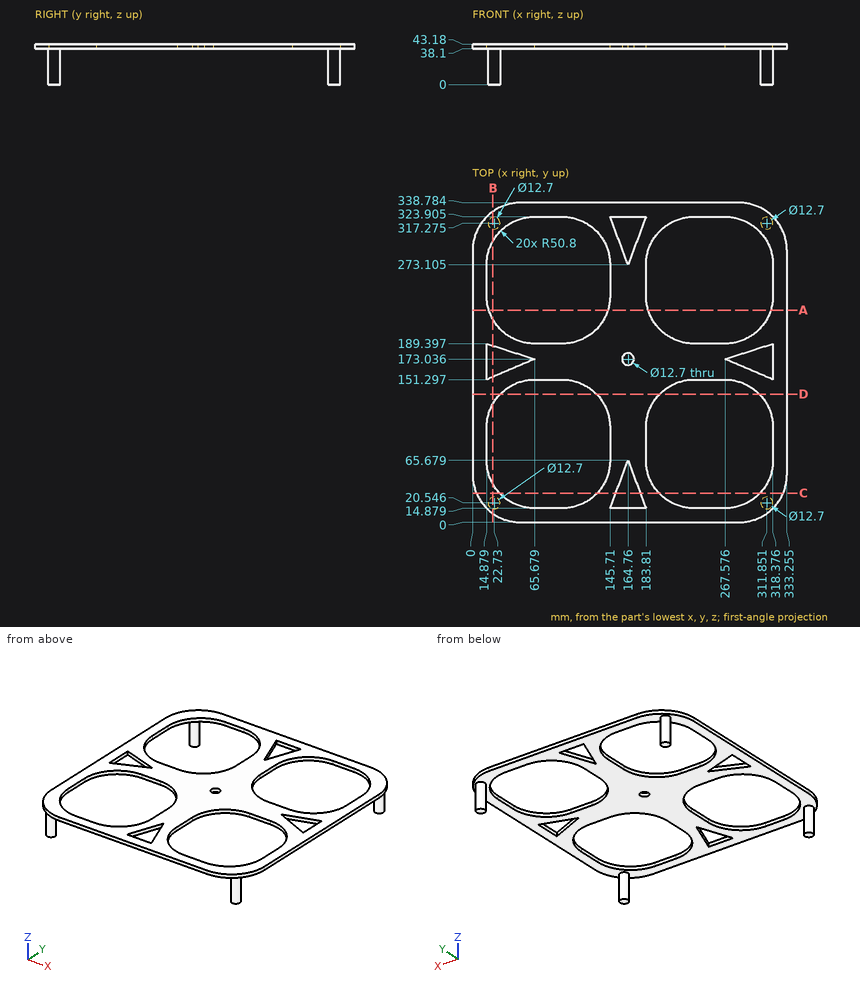
Here's the drawing with two shaded views (mm, measured from the low corner). I have some questions. Round coordinates to 2 decimals unless told otherwise and drop trailing zeros. Order: outer loops, then holes, each group sorted by start corner. A loop starts at its lowest first (then second) coordinate and runs counter-clockwise, first axis right, second up. Notation, with made-up numbers: (-4, 81.25) -> (12, 81.25) arc R14 ccw to (12, 101.25) -> close; hole circle Ø11 at (12.5, -13.75). An arc over 180 degrees is marked (long way). Use a Markdown table: item, result. Add a question column.
(1) I need wall thicknesses on line 1 along Y through (x, z) = (85.5, 40) (1 decimal); line 2 along Y through (x, z) = (300, 41) (1 decimal); line 3 along Z through (x, y) = (179, 100). Which ranges of each line are inside material? Lowest first, please.
(2) For pin 1 Ø6 at (x, y) = (187, 84.5) entering from -Z; pin 2 Ø4 at (x, y) = (250, 161.5) entering from -Z, each with a flat end and sliding along its axis, tell me the tip position at first contact or that it passes through.
(3) Suppose I cut it at A-A, the plane y = 225. Count the separate pieces of the cut face and the enclosed holes in it, and give its area (3 significant figures).
(4) Suppose I cut it at C-C, the plane y = 31. Please give me the cut outline in (x, z) (1 decimal).
(5) Suppose I cut it at D-D, the plane y = 136. Please give me the cut outline in (x, z) (1 decimal).
(6) Suppose I cut it at B-B, the plane x = 21.5. Please give me the cut outline in (y, z) (1 decimal).
Verdict:
| question | item | result |
|---|---|---|
| 1 | line 1 | 0 to 14.9, 151.3 to 189.4, 323.9 to 338.8 |
| 1 | line 2 | 3.1 to 26.6, 139.6 to 159.2, 183.5 to 201.1, 312.2 to 335.7 |
| 1 | line 3 | 38.1 to 43.18 |
| 2 | pin 1 | through |
| 2 | pin 2 | z = 38.1 |
| 3 | separate pieces | 3 |
| 3 | enclosed holes | 0 |
| 3 | area | 392 mm2 |
| 4 | outline | (4, 38.1) -> (28.6, 38.1) -> (28.6, 43.2) -> (4, 43.2) -> close; (132, 38.1) -> (151.8, 38.1) -> (151.8, 43.2) -> (132, 43.2) -> close; (177.8, 38.1) -> (197.5, 38.1) -> (197.5, 43.2) -> (177.8, 43.2) -> close; (304.7, 38.1) -> (329.2, 38.1) -> (329.2, 43.2) -> (304.7, 43.2) -> close |
| 5 | outline | (0, 38.1) -> (29.3, 38.1) -> (29.3, 43.2) -> (0, 43.2) -> close; (131.2, 38.1) -> (198.3, 38.1) -> (198.3, 43.2) -> (131.2, 43.2) -> close; (303.9, 38.1) -> (333.3, 38.1) -> (333.3, 43.2) -> (303.9, 43.2) -> close |
| 6 | outline | (9.3, 38.1) -> (14.3, 38.1) -> (14.3, 0) -> (26.8, 0) -> (26.8, 38.1) -> (40.6, 38.1) -> (40.6, 43.2) -> (9.3, 43.2) -> close; (125.6, 38.1) -> (154.1, 38.1) -> (154.1, 43.2) -> (125.6, 43.2) -> close; (187.3, 38.1) -> (215.1, 38.1) -> (215.1, 43.2) -> (187.3, 43.2) -> close; (298.2, 38.1) -> (311, 38.1) -> (311, 0) -> (323.5, 0) -> (323.5, 38.1) -> (329.5, 38.1) -> (329.5, 43.2) -> (298.2, 43.2) -> close |
